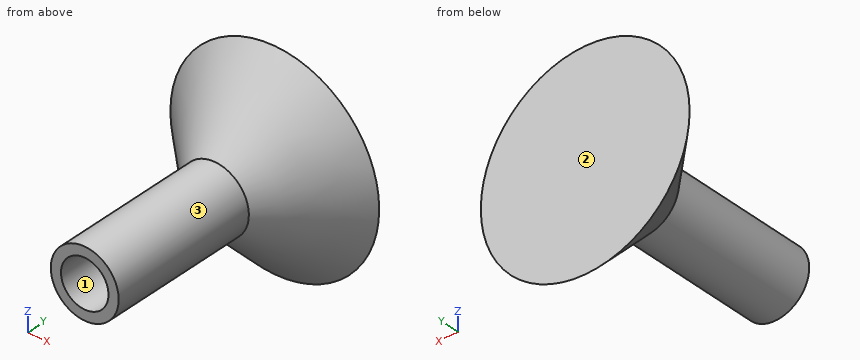
from build123d import *

# Parameters (mm, degrees)
SKETCH2_R           = 2.217157288
BOSS_EXTRUDE1_DEPTH = 10
SKETCH3_R           = 1.55
BOSS_EXTRUDE2_DEPTH = 3
SKETCH3_2_R         = 1.55
CUT_EXTRUDE1_DEPTH  = 5


with BuildPart() as part:
    # Sketch1 → Revolve1 (revolve)
    with BuildSketch(Plane.XY, mode=Mode.PRIVATE) as revolve1_sk:
        Polygon((-0.2, 2.3), (-0.2, -2.3), (-2.417157288, -2.3), (-7.017157288, 2.3), align=None)
    revolve(revolve1_sk.sketch.rotate(Axis((-0.2, 2.3, 0), (0, -1, 0)), 270), axis=Axis((-0.2, 2.3, 0), (0, -1, 0)))

    # Sketch2 → Boss-Extrude1 (add)
    with BuildSketch(Plane.XZ.offset(2.3)):
        with Locations(Location((-0.2, 0, 0), (0, 0, 90))):
            Circle(SKETCH2_R)
    extrude(amount=BOSS_EXTRUDE1_DEPTH)

    # Sketch3 → Boss-Extrude2 (add)
    with BuildSketch(Plane.XZ.offset(12.3)):
        with Locations((-0.2, 0)):
            Circle(SKETCH3_R)
    extrude(amount=-BOSS_EXTRUDE2_DEPTH)

    # Sketch3_2 → Cut-Extrude1 (cut)
    with BuildSketch(Plane.XZ.offset(12.3)):
        with Locations(Location((-0.2, 0, 0), (0, 0, 270))):
            Circle(SKETCH3_2_R)
    extrude(amount=-CUT_EXTRUDE1_DEPTH, mode=Mode.SUBTRACT)


solid = part.part
Design review of the part built by this model. Coordinates are the model's own, in mm. Face numbers are marked on the shaded views. Coordinates: 2 decimals unless noted, no trailing zeros. Loops run counter-clockwise (first coordinate to the right, second up) from the corner with the lowest first, then second, coordinate; pieces in that order, holes last. Notation, with made-up numbers: (74.5, 31.5) -> (93.5, 31.5) arc R12 cw to (93.5, 48.5) -> close; hole circle Ø6 at (76.25, 86). An arc over 180 degrees is marked (long way). Use a Markdown table: item, result. Add a question column.
Item 1: We need section C-C, the plane y = -9.5. Write out the cut boundary in (x, z).
Item 2: We need section D-D, the plane y = -4.75. Write out the cut boundary in (x, z), and give its area (3 significant figures).
Item 3: Wall thickness on L1, parallel to X at y = -9.3, z = 0; L2, parallel to Y at x = 0.5, z = 0.5; L3, parallel to X at y = -9, z = 1: over which ranges is each line inside the solid? List them lowest first. Write a range as from..to.
Item 4: We need section B-B, the plane x = -0.2. Write out the cut boundary in (y, z), and give its area (3 significant figures).
Item 5: Clearance check with flat-ended pins moving along their axes: P1, Ø8, axis at x = 1.5, y = -1, coming from the +Z side; P2, Ø1.5, axis at x = 1, y = -3.5, coming from the -Z side; P3, Ø2, axis at x = 4.5, y = -0.5, coming from the +Z side; P4, Ø2, axis at y = -9, z = -1, coming from the -X side. State where each tip first meets the part, or that it passes through.
Item 6: We need section A-A, the plane z = 0. Write out the cut boundary in (x, y), and give its area (3 significant figures).
Item 7: The part is to be moulded in two halves that separate along Z. For the marked faces 1, 2 and 3, say which applies: +Z half, -Z half, draft (parallel to the pull), parting line (faces both ways), or undercut.
Numbers:
| question | item | result |
|---|---|---|
| 1 | outline | circle Ø4.43 at (-0.2, 0); hole circle Ø3.1 at (-0.2, 0) |
| 2 | outline | circle Ø4.43 at (-0.2, 0) |
| 2 | area | 15.4 mm^2 |
| 3 | L1 | x = -2.42..-1.75, 1.35..2.02 |
| 3 | L2 | y = -7.3..2.3 |
| 3 | L3 | x = -2.18..-1.38, 0.98..1.78 |
| 4 | outline | (-12.3, -2.22) -> (-2.3, -2.22) -> (2.3, -6.82) -> (2.3, 6.82) -> (-2.3, 2.22) -> (-12.3, 2.22) -> (-12.3, 1.55) -> (-7.3, 1.55) -> (-7.3, -1.55) -> (-12.3, -1.55) -> close |
| 4 | area | 70.4 mm^2 |
| 5 | P1 | stops at z = 6.82 |
| 5 | P2 | stops at z = -2.17 |
| 5 | P3 | stops at z = 2.53 |
| 5 | P4 | stops at x = -2.42 |
| 6 | outline | (-7.02, 2.3) -> (-2.42, -2.3) -> (-2.42, -12.3) -> (-1.75, -12.3) -> (-1.75, -7.3) -> (1.35, -7.3) -> (1.35, -12.3) -> (2.02, -12.3) -> (2.02, -2.3) -> (6.62, 2.3) -> close |
| 6 | area | 70.4 mm^2 |
| 7 | face 1 | undercut |
| 7 | face 2 | draft |
| 7 | face 3 | parting line |
